Study the drawing (mm; zero at the part's minimum x, y, z) and answer. A direction names the side the tool comes from. Round coordinates to 2 decimals unless told otherwise and drop trailing zeros. Write each loop counter-clockwise with the first axis right and the second up, starting at its lowest first coordinate (ties: lowest second). Pieces come first, ordered by that corner, then holes. Notation, with made-up numbers: (16.5, 13.5) -> (25.5, 13.5) arc R33 ccw to (25.5, 47.5) -> close; hole circle Ø8 at (56.5, -7.75). An arc over 180 degrees is marked (long way). One line per question, with ' | ' between items. Start each with the question number.
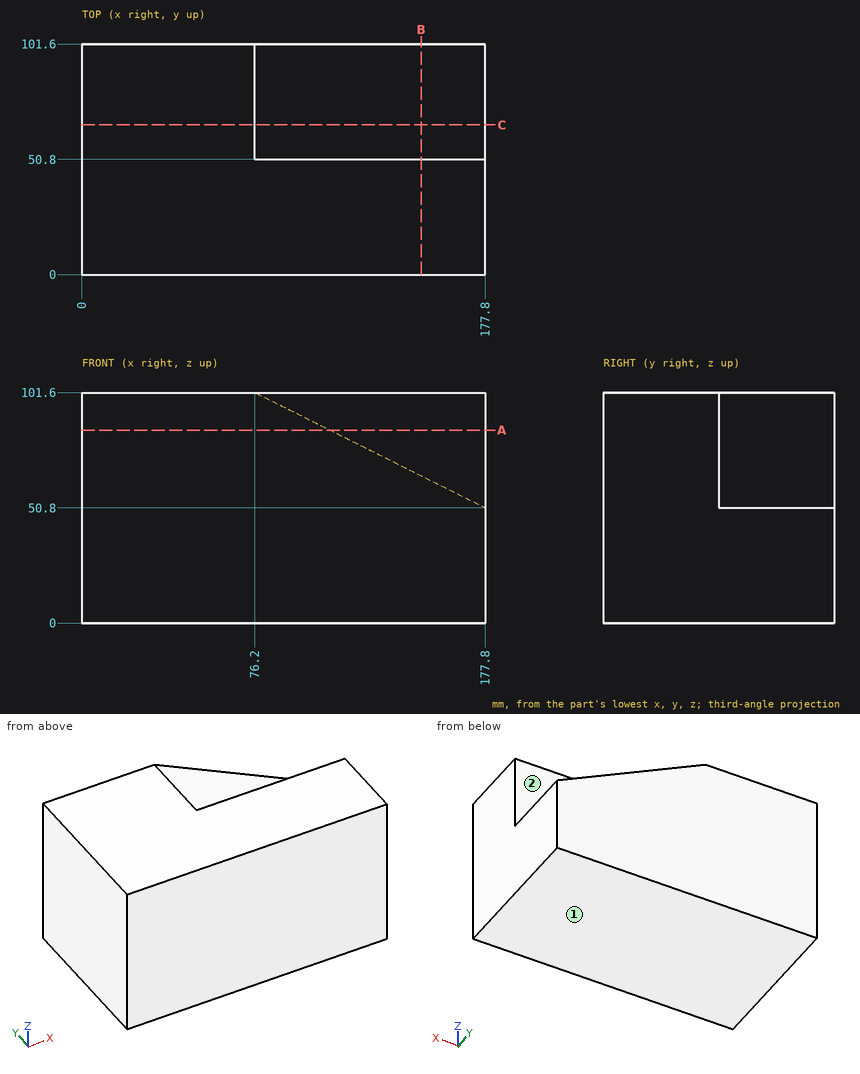
(1) Consider L1, parallel to Y at x = 118.5, z = 92.5; L2, parallel to Z at x = 102, y = 79; L3, parallel to Z at x = 137, y = 53. Determine where each line is inside the solid, lowest interval first.
(2) A cutting plane is placed at B-B, the plane x = 149.5. Determine the outline of the cut face in (y, z).
(3) A cutting plane is placed at A-A, the plane z = 85. Determine the outline of the cut face in (x, y).
(4) For the marked faces 1 and 2, determine the directions among +Z, -Z, +X, -X, +Y, -Y from which every point of the face is accessible in a straight line to the end or side of a thin tool.
(5) A cutting plane is placed at C-C, the plane y = 66. Determine the outline of the cut face in (x, z), then the cut area to 3 significant figures.
(6) Given pin 1 Ø8 at (x, y) = (110.5, 90.5) entering from +Z; pin 2 Ø4 at (x, y) = (81.5, 70) entering from +Z; pin 3 Ø15 at (x, z) = (143, 88.5) entering from +Y, each flat-ended and moving along its own axis, determine where each tip first touches the part or whether it passes through.
Returned:
1) L1: 0 to 50.8 | L2: 0 to 88.7 | L3: 0 to 71.2
2) outline: (0, 0) -> (101.6, 0) -> (101.6, 64.95) -> (50.8, 64.95) -> (50.8, 101.6) -> (0, 101.6) -> close
3) outline: (0, 0) -> (177.8, 0) -> (177.8, 50.8) -> (109.4, 50.8) -> (109.4, 101.6) -> (0, 101.6) -> close
4) face 1: -Z, +X, -X, +Y, -Y | face 2: +Z, +X, +Y
5) outline: (0, 0) -> (177.8, 0) -> (177.8, 50.8) -> (76.2, 101.6) -> (0, 101.6) -> close | area: 15,500 mm2
6) pin 1: z = 86.45 | pin 2: z = 99.95 | pin 3: y = 50.8
